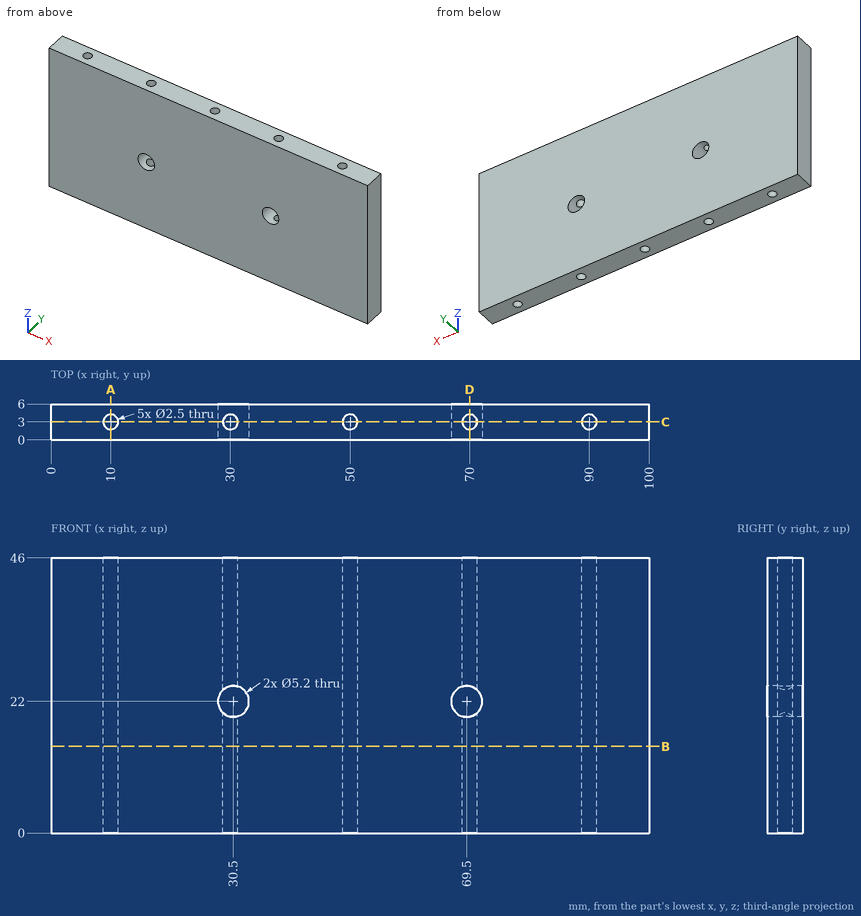
Study the drawing (mm; zero at the part's minimum x, y, z) and answer. Give positions to 0.01 mm unless a question says otherwise; leave off trailing zeros. Order: outer loops, then holes, each group sorted by start corner. A loop starts at its lowest first (then second) coordinate and runs counter-clockwise, first axis right, second up. Notation, with made-up numbers: (-8, -38) - (34, -38) arc R32 ccw to (34, -11) - close; hole circle Ø9 at (37, -27). An arc over 180 degrees is marked (long way). Answer in a Markdown table with one row per item. Add a question column.
Q1. Find the intervals of material crossed by line 1 along Y through (x, z) = (70, 31); line 2 along X through (y, z) = (3.75, 9); line 3 along X through (y, z) = (3.5, 27), in increasing order. Write a range as [from, to].
Q2. The part is cut by section B-B (z = 14.5). Determine the outline of the cut face in (x, y).
Q3. The part is cut by section A-A (x = 10). Determine the outline of the cut face in (y, z).
Q4. The part is cut by section D-D (x = 70). Determine the outline of the cut face in (y, z), then the cut area to 3 significant figures.
Q5. The part is cut by section C-C (y = 3). Give the number of separate pieces and of enclosed holes in the cut face, then the cut area to 3 significant figures.
Determined:
| question | item | result |
|---|---|---|
| 1 | line 1 | y = [0, 1.75], [4.25, 6] |
| 1 | line 2 | x = [0, 9], [11, 29], [31, 49], [51, 69], [71, 89], [91, 100] |
| 1 | line 3 | x = [0, 8.85], [11.15, 28.85], [31.15, 48.85], [51.15, 68.85], [71.15, 88.85], [91.15, 100] |
| 2 | outline | (0, 0) - (100, 0) - (100, 6) - (0, 6) - close; hole circle Ø2.5 at (10, 3); hole circle Ø2.5 at (30, 3); hole circle Ø2.5 at (50, 3); hole circle Ø2.5 at (70, 3); hole circle Ø2.5 at (90, 3) |
| 3 | outline | (0, 0) - (1.75, 0) - (1.75, 46) - (0, 46) - close; (4.25, 0) - (6, 0) - (6, 46) - (4.25, 46) - close |
| 4 | outline | (0, 0) - (1.75, 0) - (1.75, 19.45) - (0, 19.45) - close; (0, 24.55) - (1.75, 24.55) - (1.75, 46) - (0, 46) - close; (4.25, 0) - (6, 0) - (6, 19.45) - (4.25, 19.45) - close; (4.25, 24.55) - (6, 24.55) - (6, 46) - (4.25, 46) - close |
| 4 | area | 143 mm² |
| 5 | separate pieces | 6 |
| 5 | enclosed holes | 0 |
| 5 | area | 4,010 mm² |
